Here's the drawing with two shaded views (mm, measured from the low corner). I have some questions. A direction names the side the tool comes from. Round coordinates to 2 decimals unless told otherwise and drop trailing zeros. Loops run counter-clockwise (first coordinate to the right, second up) from the corner with the lowest first, then second, coordinate; pieces in that order, holes last.
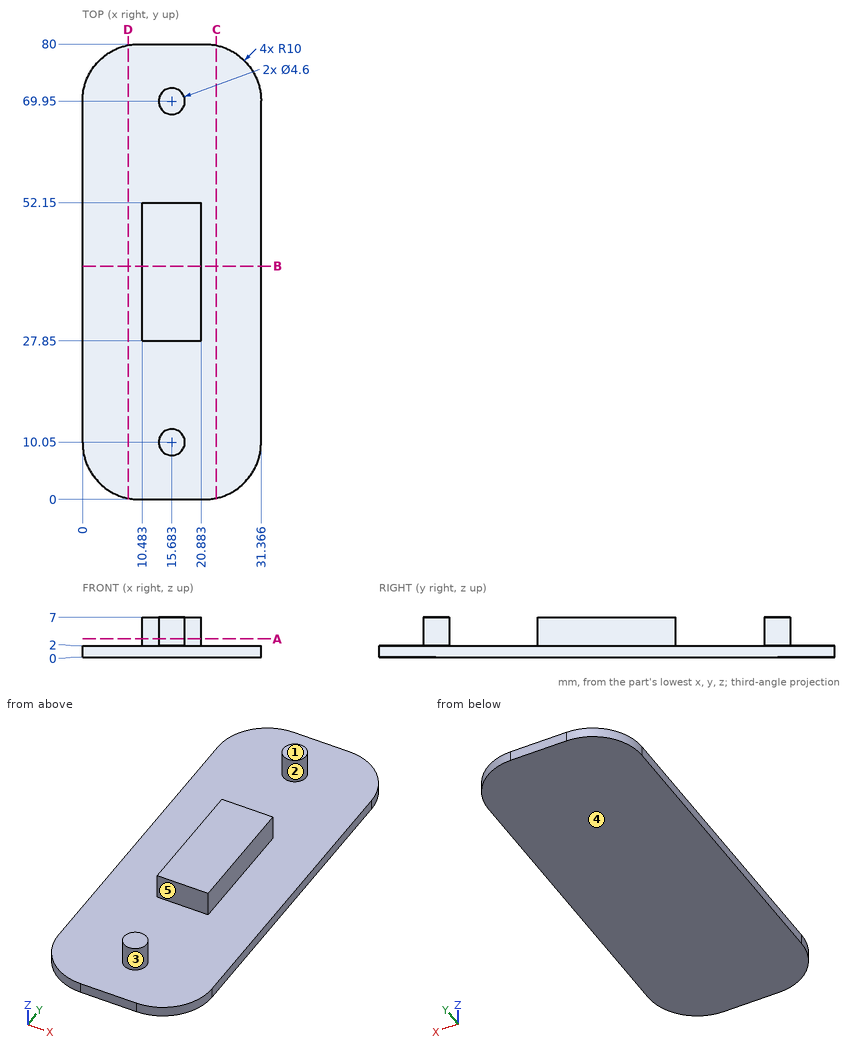
Item 1: If we section it at D-D, the plane x = 8: Please give me the cut outline in (y, z), then the cut area to 3 significant figures.
Results list:
outline: (0.2, 0) - (79.8, 0) - (79.8, 2) - (0.2, 2) - close
area: 159 mm2
Item 2: For the marked faces 3, 4 and 5, which set-ups out of +Z, -Z, +X, -X, +Y, -Y let a thin tool reach every point of the face, with its end or its side?
Results list:
face 3: +Z
face 4: -Z, +X, -X, +Y, -Y
face 5: +Z, +X, -X
Item 3: We'd pull the mould along Y, two halves only. Please class the marked faces 1 and 2: released by +Y, released by -Y, zero draft, split by the parting line, or undercut.
Results list:
face 1: zero draft
face 2: undercut
Item 4: If I drill on line 1 along Y through (x, z) = (12, 4.5); line 2 along X through (y, z) = (50, 2.5); line 3 along Y through (x, z) = (16, 3.5), over which ranges is the centre line in solid material (lowest first)?
Results list:
line 1: y = 27.85 to 52.15
line 2: x = 10.48 to 20.88
line 3: y = 7.77 to 12.33, 27.85 to 52.15, 67.67 to 72.23
Item 5: If we section it at A-A, the plane z = 3.25: Please give me the cut outline in (x, y).
Results list:
outline: (10.48, 27.85) - (20.88, 27.85) - (20.88, 52.15) - (10.48, 52.15) - close; circle Ø4.6 at (15.68, 10.05); circle Ø4.6 at (15.68, 69.95)
Item 6: Will these pins go through, and if not, where does the flat tip stop? pin 1 (1.5 mm diameter, centred on y = 39, z = 4, fed in from -X); pin 2 (2.5 mm diameter, centred on x = 14.5, z = 4, fed in from +Y); pin 3 (2 mm diameter, centred on x = 9, z = 4, fed in from -Y); pin 4 (4 mm diameter, centred on x = 27.5, y = 24.5, fed in from +Z).
Results list:
pin 1: stops at x = 10.48
pin 2: stops at y = 72.25
pin 3: passes through
pin 4: stops at z = 2
Item 7: If we section it at B-B, the plane y = 41: Please give me the cut outline in (x, z).
Results list:
outline: (0, 0) - (31.37, 0) - (31.37, 2) - (20.88, 2) - (20.88, 7) - (10.48, 7) - (10.48, 2) - (0, 2) - close
Item 8: If we section it at C-C, the plane x = 23.5: Please give me the cut outline in (y, z).
Results list:
outline: (0.23, 0) - (79.77, 0) - (79.77, 2) - (0.23, 2) - close
